The model under review builds one solid part; all positions refer to its coordinate system, in mm. Face numbers are marked on the shaded views. A direction names the side the tool comes from. Give positions to 0.01 mm unless a question says otherwise; leave off trailing zeros. Loops run counter-clockwise (first coordinate to the right, second up) from the corner with the lowest first, then second, coordinate; pieces in that order, holes last. Notation, with made-up numbers: M -19.75,27 L 14.25,27 A20 cw 14.25,56 Z; hole C 70.5,6.5 d4. An arc over 180 degrees is marked long. Return JSON: item names as keys, results as strings.
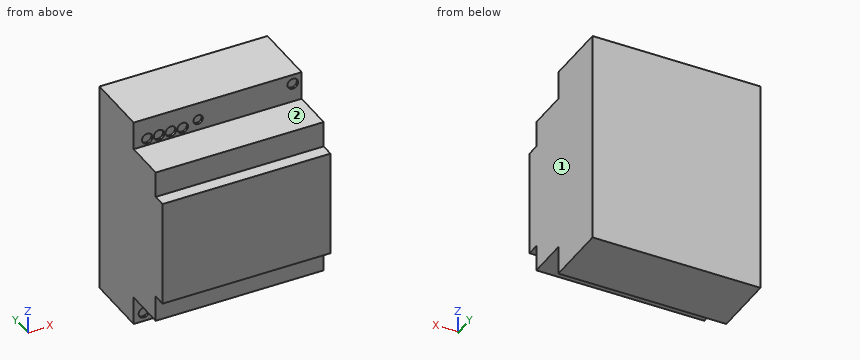
```python
from build123d import *

# Parameters (mm, degrees)
F0_W     = 71
F0_H     = 91
F1_DEPTH = 50
F2_W     = 71
F2_H     = 12
F3_DEPTH = 22.9
F4_W     = 71
F4_H     = 11
F5_DEPTH = 5.4
F6_R     = 2.25
F6_R_2   = 2
F7_DEPTH = 1


with BuildPart() as f1:
    # F0 (on Front) → F1 (new body)
    with BuildSketch(Plane.XZ):
        Rectangle(F0_W, F0_H)
    extrude(amount=F1_DEPTH)

    # F2 (on face) → F3 (cut)
    with BuildSketch(Plane.XZ.offset(50)):
        with Locations((0, 39.5)):
            Rectangle(F2_W, F2_H)
        with Locations((0, -39.5)):
            Rectangle(F2_W, F2_H)
    extrude(amount=-F3_DEPTH, mode=Mode.SUBTRACT)

    # F4 (on face) → F5 (cut)
    with BuildSketch(Plane.XZ.offset(50)):
        with Locations((0, 28)):
            Rectangle(F4_W, F4_H)
        with Locations((0, -28)):
            Rectangle(F4_W, F4_H)
    extrude(amount=-F5_DEPTH, mode=Mode.SUBTRACT)

    # F6 (on face) → F7 (cut)
    with BuildSketch(Plane.XZ.offset(27.1)):
        with Locations((-29.748868, 36.449973)):
            Circle(F6_R)
        with Locations((-24.748868, 36.449973)):
            Circle(F6_R)
        with Locations((-19.748868, 36.449973)):
            Circle(F6_R)
        with Locations((-14.748868, 36.449973)):
            Circle(F6_R)
        with Locations((-8.246585, 38.107269)):
            Circle(F6_R_2)
        with Locations((31.766169, 41.469164)):
            Circle(F6_R)
        with Locations((-31.138731, -41.702226)):
            Circle(F6_R)
        with Locations((20.723933, -36.418043)):
            Circle(F6_R)
        with Locations((31.085899, -36.418043)):
            Circle(F6_R)
    extrude(amount=-F7_DEPTH, mode=Mode.SUBTRACT)


solid = f1.part
```
1) Tool access review of the marked faces 1 and 2: name each direction out of +Z, -Z, +X, -X, +Y, -Y from which nothing blocks a thin tool from reaching the whole face with its end or side.
From the geometry:
{"face 1": "+Z, -Z, +X, +Y, -Y", "face 2": "+Z, +X, -X, -Y"}
2) Consider section B-B on y = -40.5. Write out the cut boundary in (x, z).
From the geometry:
{"outline": "M -35.5,-33.5 L 35.5,-33.5 L 35.5,33.5 L -35.5,33.5 Z"}
3) Consider section A-A on x = 0. Write out the cut boundary in (y, z).
From the geometry:
{"outline": "M -50,-22.5 L -44.6,-22.5 L -44.6,-33.5 L -27.1,-33.5 L -27.1,-45.5 L 0,-45.5 L 0,45.5 L -27.1,45.5 L -27.1,33.5 L -44.6,33.5 L -44.6,22.5 L -50,22.5 Z"}
4) Insertion check: pin 1 (10 mm diameter, centred on x = 3, y = -37, fed in from +Z); pin 2 (9 mm diameter, centred on x = -5, z = -30, fed in from -Y); pin 3 (3.5 mm diameter, centred on x = 21.5, z = -36.5, fed in from -Y). Each pin has a flat end and moves straight along its axis. Give the tip position at first contact, or say it passes through.
From the geometry:
{"pin 1": "z = 33.5", "pin 2": "y = -44.6", "pin 3": "y = -27.1"}
5) Consider section D-D on x = -9. Write out the cut boundary in (y, z), then the cut area to 3 significant figures.
From the geometry:
{"outline": "M -50,-22.5 L -44.6,-22.5 L -44.6,-33.5 L -27.1,-33.5 L -27.1,-45.5 L 0,-45.5 L 0,45.5 L -27.1,45.5 L -27.1,39.96 L -26.1,39.96 L -26.1,36.25 L -27.1,36.25 L -27.1,33.5 L -44.6,33.5 L -44.6,22.5 L -50,22.5 Z", "area": "3,880 mm²"}
6) Consider section C-C on z = -30. Write out the cut boundary in (x, y), then the cut area to 3 significant figures.
From the geometry:
{"outline": "M -35.5,-44.6 L 35.5,-44.6 L 35.5,0 L -35.5,0 Z", "area": "3,170 mm²"}
7) Wall thickness on L1, parallel to Z at x = -31.5, y = -43; L2, parallel to Y at x = 17.5, z = -29.5; L3, parallel to Z at x = 26.5, y = -47: over which ranges is each line inside the solid? List them lowest first. Write a range as from..to.
From the geometry:
{"L1": "-33.5..33.5", "L2": "-44.6..0", "L3": "-22.5..22.5"}
